Work out the finished part from the listing and answer in its coordinate system (mm). Face numbers are marked on the shaded views. Give positions to 0.01 mm unless a question says otherwise; leave off trailing zeros. Write each loop counter-clockwise with the first axis right and the second up, starting at its lowest first coordinate (ties: lowest second). Pieces come first, ordered by that corner, then holes.
1) Find section B-B (z = 4). Count the separate pieces of the cut face and the enclosed holes in it, plus the area to 3 significant figures.
2) Straight lines are drawn through the part: probe 1 along Z at (x, y) = (0, 47.8); probe 2 along Y at (x, z) = (-30, 4.75); probe 3 along X at (y, z) = (-2.5, 4). For each, find the intervals that lie inside material, in ascending order.
3) Find section D-D (y = 13). Determine the outline of the cut face in (x, z), plus the area to 3 significant figures.
4) Find section C-C (x = 30). Determine the outline of the cut face in (y, z), plus the area to 3 significant figures.
5) Given pin 1 Ø1.8 at (y, z) = (0, 4) entering from -X; pin 2 Ø2 at (y, z) = (-15.5, 2.5) entering from -X; pin 3 Ø4 at (x, z) = (27.5, 7) entering from -Y; pin 4 Ø1.2 at (x, y) = (14, 7.5) entering from +Z, each flat-ended and moving along its own axis, determine where each tip first touches the part or whether it passes through.
6) Find section A-A (x = 0). Determine the outline of the cut face in (y, z), plus the area to 3 significant figures.
7) Determine the mould class of the marked faces 1, 2 and 3 for opening direction X: pulls with the +X half, pulls with the -X half, needs draft (parallel to the pull), parting line crosses it, or undercut.
Autodesk Inventor part; units mm, degrees
ref_plane "作業平面1" through (50, 0, 0) normal (1, 0, 0) x (0, 1, 0)
ref_plane "作業平面2" through (-50, 0, 0) normal (1, 0, 0) x (0, 1, 0)
ref_plane "作業平面3" through (0, 50, 0) normal (0, 1, 0) x (-1, 0, 0)
sketch "スケッチ1" plane through (0, 0, 0) normal (0, 0, 1) x (1, 0, 0)
  circle A0 centre (0, 0) radius 50
  dimension "d0" = 100
extrude "押し出し1" add sketch "スケッチ1" along normal blind 8
ref_plane "作業平面1" through (50, 0, 0) normal (1, 0, 0) x (0, 1, 0)
ref_plane "作業平面2" through (-50, 0, 0) normal (1, 0, 0) x (0, 1, 0)
ref_plane "作業平面3" through (0, 50, 0) normal (0, 1, 0) x (-1, 0, 0)
ref_plane "作業平面4" through (0, -50, 0) normal (0, 1, 0) x (-1, 0, 0)
sketch "スケッチ2" plane through (50, 0, 0) normal (1, 0, 0) x (0, 1, 0)
  line L0 (0, 0) -> (0, 4) construction
  circle A0 centre (0, 4) radius 1.5
  dimension "d7" = 4
  dimension "d8" = 3
extrude "押し出し2" cut sketch "スケッチ2" against normal blind 5
sketch "スケッチ3" plane through (-50, 0, 0) normal (1, 0, 0) x (0, 1, 0)
  line L0 (0, 0) -> (0, 4) construction
  circle A0 centre (0, 4) radius 1.5
  dimension "d11" = 4
  dimension "d12" = 3
extrude "押し出し3" cut sketch "スケッチ3" along normal blind 5
sketch "スケッチ4" plane through (0, 50, 0) normal (0, 1, 0) x (-1, 0, 0)
  line L0 (0, 0) -> (0, 4) construction
  circle A0 centre (0, 4) radius 1.5
  dimension "d15" = 4
  dimension "d16" = 3
extrude "押し出し4" cut sketch "スケッチ4" against normal blind 5
sketch "スケッチ5" plane through (0, -50, 0) normal (0, 1, 0) x (-1, 0, 0)
  line L0 (0, 0) -> (0, 4) construction
  circle A0 centre (0, 4) radius 1.5
  dimension "d19" = 4
  dimension "d20" = 3
extrude "押し出し5" cut sketch "スケッチ5" along normal blind 5
thread "ねじ1"
thread "ねじ2"
thread "ねじ3"
thread "ねじ4"
sketch "スケッチ8" plane through (0, 0, 8) normal (0, 0, 1) x (1, 0, 0)
  line L0 (0, 0) -> (0, 18.5) construction
  line L1 (0, 0) -> (0, -18.5) construction
  circle A0 centre (0, 18.5) radius 2
  circle A1 centre (0, -18.5) radius 2
  circle A2 centre (0, 0) radius 6.5
  dimension "d62" = 18.5
  dimension "d63" = 18.5
  dimension "d64" = 4
  dimension "d65" = 4
  dimension "d66" = 13
extrude "押し出し7" cut sketch "スケッチ8" against normal blind 8
thread "ねじ7"
thread "ねじ8"
sketch "スケッチ9" plane through (0, 0, 8) normal (0, 0, 1) x (1, 0, 0)
  line L0 (0, 0) -> (25, 0) construction
  line L1 (25, 0) -> (25, -1) construction
  line L2 (25, 0) -> (25, 7.5) construction
  circle A0 centre (36, 7.5) radius 1
  line L3 (36, 7.5) -> (14, 7.5) construction
  circle A1 centre (14, 7.5) radius 1
  line L4 (25, -1) -> (25, -10) construction
  line L5 (25, -10) -> (25, -28) construction
  circle A2 centre (11.5, -28) radius 1
  line L6 (25, 0) -> (9, 0) construction
  line L7 (9, 0) -> (9, -31) construction
  line L8 (9, -31) -> (41, -31) construction
  line L9 (41, -31) -> (41, 0) construction
  line L10 (25, 0) -> (25, 12) construction
  line L11 (14.417, 12) -> (35.583, 12) construction
  arc A3 (14.757, 12.2915) -> (9, 0) centre (25, 0) ccw construction
  arc A4 (41, 0) -> (35.583, 12) centre (25, 0) ccw construction
  line L12 (11.5, -28) -> (38.5, -28) construction
  circle A5 centre (38.5, -28) radius 1
  dimension "d92" = 25
  dimension "d103" = 7.5
  dimension "d105" = 2
  dimension "d108" = 2
  dimension "d117" = 2
  dimension "d129" = 16
  dimension "d130" = 31
  dimension "d131" = 32
  dimension "d134" = 22
  dimension "d146" = 28
  dimension "d147" = 27
  dimension "d148" = 2
sketch "スケッチ10" plane through (0, 0, 8) normal (0, 0, 1) x (1, 0, 0)
  line L0 (0, 0) -> (-25, 0) construction
  line L1 (-35.65, 22.85) -> (-14.35, 22.85) construction
  line L2 (-14.35, 22.85) -> (-14.35, -22.85) construction
  line L3 (-14.35, -22.85) -> (-35.65, -22.85) construction
  line L4 (-35.65, -22.85) -> (-35.65, 22.85) construction
  line L5 (-35.65, 22.85) -> (-14.35, -22.85) construction
  line L6 (-14.35, 22.85) -> (-35.65, -22.85) construction
  line L7 (-35.65, 22.85) -> (-32.15, 22.85) construction
  line L8 (-32.15, 22.85) -> (-32.15, 19.35) construction
  line L9 (-32.15, 19.35) -> (-35.65, 19.35) construction
  line L10 (-35.65, 19.35) -> (-35.65, 22.85) construction
  line L11 (-14.35, -22.85) -> (-17.85, -22.85) construction
  line L12 (-17.85, -22.85) -> (-17.85, -19.35) construction
  line L13 (-17.85, -19.35) -> (-14.35, -19.35) construction
  line L14 (-14.35, -19.35) -> (-14.35, -22.85) construction
  circle A0 centre (-32.15, 19.35) radius 1.5
  circle A1 centre (-17.85, -19.35) radius 1.5
  dimension "d135" = 25
  dimension "d136" = 21.3
  dimension "d137" = 45.7
  dimension "d138" = 3.5
  dimension "d139" = 3.5
  dimension "d140" = 3.5
  dimension "d141" = 3.5
  dimension "d142" = 3
  dimension "d143" = 3
extrude "押し出し10" cut sketch "スケッチ10" against normal blind 8
extrude "押し出し11" cut sketch "スケッチ9" against normal blind 8
sketch "スケッチ13" plane through (0, 0, 8) normal (0, 0, 1) x (1, 0, 0)
  line L0 (0, 0) -> (-35, 0) construction
  line L1 (-40, 5) -> (-30, 5) construction
  line L2 (-30, 5) -> (-30, -5) construction
  line L3 (-30, -5) -> (-40, -5) construction
  line L4 (-40, -5) -> (-40, 5) construction
  line L5 (-40, 5) -> (-30, -5) construction
  line L6 (-30, 5) -> (-40, -5) construction
  circle A0 centre (-30, 5) radius 1
  circle A1 centre (-30, -5) radius 1
  circle A2 centre (-40, 5) radius 1
  circle A3 centre (-40, -5) radius 1
  dimension "d151" = 35
  dimension "d152" = 10
  dimension "d153" = 10
  dimension "d154" = 2
  dimension "d155" = 2
  dimension "d156" = 2
  dimension "d157" = 2
extrude "押し出し12" cut sketch "スケッチ13" against normal blind 8
properties part number "outsideCover"
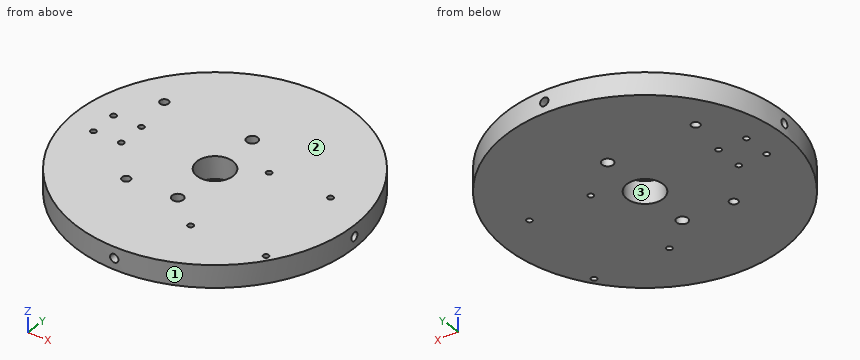
Results:
1. separate pieces: 1
1. enclosed holes: 13
1. area: 7,600 mm2
2. probe 1: z = 0 to 2.5, 5.5 to 8
2. probe 2: y = -40 to -6, -4 to 4, 6 to 40
2. probe 3: x = -49.94 to -6, 6 to 49.94
3. outline: (-48.28, 0) - (48.28, 0) - (48.28, 8) - (-48.28, 8) - close
3. area: 772 mm2
4. outline: (-40, 0) - (40, 0) - (40, 8) - (-40, 8) - close
4. area: 640 mm2
5. pin 1: stops at x = -45
5. pin 2: stops at x = -47.85
5. pin 3: stops at y = -43.01
5. pin 4: passes through
6. outline: (-50, 0) - (-20.5, 0) - (-20.5, 8) - (-50, 8) - (-50, 5.5) - (-45, 5.5) - (-45, 2.5) - (-50, 2.5) - close; (-16.5, 0) - (-6.5, 0) - (-6.5, 8) - (-16.5, 8) - close; (6.5, 0) - (16.5, 0) - (16.5, 8) - (6.5, 8) - close; (20.5, 0) - (50, 0) - (50, 2.5) - (45, 2.5) - (45, 5.5) - (50, 5.5) - (50, 8) - (20.5, 8) - close
6. area: 602 mm2
7. face 1: parting line crosses it
7. face 2: needs draft
7. face 3: undercut
